Geometry: final body of the model. Coordinates: model frame, mm. A direction names the side the tool comes from. Give positions to 0.01 mm unless a question says otherwise; leave off trailing zeros. Loops run counter-clockwise (first coordinate to the right, second up) from the corner with the lowest first, then second, coordinate; pieces in that order, holes last. Notation, with made-up numbers: (3, 84) - (13, 84) arc R33 cw to (13, 118) - close; hole circle Ø6 at (44.25, -7). An arc over 180 degrees is marked (long way). Answer in a Markdown table with one row per item.
from build123d import *

# Parameters (mm, degrees)
F2_DEPTH = 2.5
F3_R     = 5
F4_R     = 1


with BuildPart() as f1:
    # F0 (on Top) → F1 (revolve)
    with BuildSketch(Plane.XY):
        Polygon((17, 83.3376), (0, 83.3376), (0, 53.3376), (7, 53.3376), (17, 53.3376), align=None)
    revolve(axis=Axis((0, 2.958108, 0), (0, -1, 0)))

    # F0 (on Top) → F2 (join, symmetric)
    with BuildSketch(Plane.XY):
        with BuildLine():
            Line((7, 53.3376), (0, 53.3376))
            Line((0, 53.3376), (0, -16.6624))
            ThreePointArc((0, -16.6624), (3, -19.6624), (0, -22.6624))
            Line((0, -22.6624), (0, -26.6624))
            Line((0, -26.6624), (7, -26.6624))
            Line((7, -26.6624), (7, 53.3376))
        make_face()
        with BuildLine():
            Line((0, -16.6624), (0, 53.3376))
            Line((0, 53.3376), (-7, 53.3376))
            Line((-7, 53.3376), (-7, -26.6624))
            Line((-7, -26.6624), (0, -26.6624))
            Line((0, -26.6624), (0, -22.6624))
            ThreePointArc((0, -22.6624), (-3, -19.6624), (0, -16.6624))
        make_face()
    extrude(amount=F2_DEPTH, both=True)

    # F3
    f3_edges = [f1.edges().sort_by_distance(p)[0] for p in [
        (7, -26.6624, 0),
        (-7, -26.6624, 0),
    ]]
    fillet(f3_edges, radius=F3_R)

    # F4
    f4_edges = [f1.edges().sort_by_distance(p)[0] for p in [
        (-17, 83.3376, 0),
    ]]
    fillet(f4_edges, radius=F4_R)


solid = f1.part
Q1. Material intervals for line 1 along Y through (x, z) = (0, 1.3); line 2 along Y through (x, z) = (0.5, -13); line 3 along Z through (x, y) = (2.5, 1), sorted ascending.
Check values:
| item | result |
|---|---|
| line 1 | -26.66 to -22.66, -16.66 to 83.34 |
| line 2 | 53.34 to 83.34 |
| line 3 | -2.5 to 2.5 |
Q2. Cut plane B-B (z = 0). Output: boundary loops of the cut face in (x, y), and give its area (3 significant figures).
Check values:
| item | result |
|---|---|
| outline | (-17, 53.34) - (-7, 53.34) - (-7, -21.66) arc R5 ccw to (-2, -26.66) - (2, -26.66) arc R5 ccw to (7, -21.66) - (7, 53.34) - (17, 53.34) - (17, 82.34) arc R1 ccw to (16, 83.34) - (-16, 83.34) arc R1 ccw to (-17, 82.34) - close; hole circle Ø6 at (0, -19.66) |
| area | 2,100 mm² |
Q3. Cut plane C-C (y = 43). Output: boundary loops of the cut face in (x, z).
Check values:
| item | result |
|---|---|
| outline | (-7, -2.5) - (7, -2.5) - (7, 2.5) - (-7, 2.5) - close |
Q4. Reachability of faces 5 (the flat face through (0, 14, -2.5)), 6 (the cylindrical face through (-5.574, -25.159, 0.035)), 7 (the flat face through (7, 15, 0)), 8 (the flat face through (0, 14, 2.5)) from +Z, -Z, +X, -X, +Y, -Y: full face, straight path, thin tool, end or side. Return the list, or none.
Check values:
| item | result |
|---|---|
| face 5 | -Z, +X, -X, -Y |
| face 6 | +Z, -Z, -X, -Y |
| face 7 | +Z, -Z, +X, -Y |
| face 8 | +Z, +X, -X, -Y |
Q5. Cut plane D-D (y = 72.5). Output: boundary loops of the cut face in (x, z).
Check values:
| item | result |
|---|---|
| outline | circle Ø34 at (0, 0) |
Q6. Cut plane A-A (x = 0). Output: boundary loops of the cut face in (y, z).
Check values:
| item | result |
|---|---|
| outline | (-26.66, -2.5) - (-22.66, -2.5) - (-22.66, 2.5) - (-26.66, 2.5) - close; (-16.66, -2.5) - (53.34, -2.5) - (53.34, -17) - (82.34, -17) arc R1 ccw to (83.34, -16) - (83.34, 16) arc R1 ccw to (82.34, 17) - (53.34, 17) - (53.34, 2.5) - (-16.66, 2.5) - close |
Q7. Draft query along Y for faces 1 (the flat face through (0, 83.338, 0)), 2 (the flat face through (0, -26.662, 0)), 3 (the flat face through (-7, 16, 0)), 4 (the cylindrical face through (-0.132, -16.665, 0.035)). Return one class per face: pulls with the +Y half, pulls with the -Y half, needs draft (parallel to the pull), parting line crosses it, or undercut.
Check values:
| item | result |
|---|---|
| face 1 | pulls with the +Y half |
| face 2 | pulls with the -Y half |
| face 3 | needs draft |
| face 4 | undercut |
Q8. First-contact query: pin 1 (10 mm diameter, centred on x = 12.5, y = 24, fed in from +Z); pin 2 (5.5 mm diameter, centred on y = 29.5, z = -1, fed in from -X); pin 3 (1 mm diameter, centred on x = -3.5, z = -11.5, fed in from -Y); pin 4 (4 mm diameter, centred on y = 8.5, z = 0.5, fed in from +X). Flat tips, straight axial feed; report the tip coordinate or a pass-through.
Check values:
| item | result |
|---|---|
| pin 1 | through |
| pin 2 | x = -7 |
| pin 3 | y = 53.34 |
| pin 4 | x = 7 |
